```python
from build123d import *

# Parameters (mm, degrees)
F0_R     = 6
F1_DEPTH = 35
F3_DEPTH = 12.5
F5_DEPTH = 25


with BuildPart() as f1:
    # F0 (on Top) → F1 (new body)
    with BuildSketch(Plane.XY):
        Circle(F0_R)
    extrude(amount=F1_DEPTH)

    # F2 (on Front) → F3 (cut, symmetric)
    with BuildSketch(Plane.XZ):
        Polygon((6.1246007681, 35.0653016331), (-6.0470434837, 35.0653016331), (6.1246007681, 22.8936616331), align=None)
    extrude(amount=F3_DEPTH, both=True, mode=Mode.SUBTRACT)

    # F4 (on face) → F5 (join)
    with BuildSketch(Plane(origin=(14.5091301309, 0, 14.5091351992), x_dir=(0.7071069047, 0, -0.7071066577), z_dir=(0.7071066577, 0, 0.7071069047))):
        with BuildLine():
            ThreePointArc((-20.519004735, -6), (-16.2763642357, -4.2426405844), (-14.5190050255, 0))
            ThreePointArc((-14.5190050255, 0), (-16.2763643803, 4.242640729), (-20.519005144, 6))
            ThreePointArc((-20.519005144, 6), (-26.5190050255, -2.045e-07), (-20.519004735, -6))
        make_face()
    extrude(amount=F5_DEPTH)


solid = f1.part
```
Geometry check sheet. Reference: the model listing, model coordinates, mm. Coordinates: 2 decimals unless noted, no trailing zeros. Write each loop counter-clockwise with the first axis right and the second up, starting at its lowest first coordinate (ties: lowest second). Pieces come first, ordered by that corner, then holes. Notation, with made-up numbers: M 49,37.25 L 91,37.25 A28 ccw 91,76.25 Z; hole C -26,50 d2. An arc over 180 degrees is marked long. One line per item, written item: value. Start each with the question number.
(1) Sectioned sample at B-B, the plane z = 9.5. Enter the section's corners in (x, y), and give its area (3 significant figures).
(2) Sectioned sample at A-A, the plane y = -5. Enter the section's corners in (x, z), and give its area (3 significant figures).
(3) Depth check by flat-ended pin: pin 1 (5 mm diameter, centred on y = 0, z = 22, fed in from +X); pin 2 (1 mm diameter, centred on y = -3, z = 9, fed in from -X); pin 3 (4 mm diameter, centred on y = 3, z = 15, fed in from +X). Enter the tip coordinate at first touch or a pass-through.
(4) Release check for a two-part mould opening along X. For faces 1 (the face through (-4.556, -0.472, 33.574)), 2 (the face through (4.54, -0.47, 24.48)), 3 (the face through (0, 0, 0)), 4 (the face through (-6, 0, 13)) record: released by +X, released by -X, zero draft, split by the parting line, or undercut.
(5) Scan lines: line 1 along Z through (x, y) = (-4.5, 0); line 2 along Z through (x, y) = (6.75, 1.5); line 3 along X through (y, z) = (-3, 12.5). Record each from-to range of solid material in increasing order. Write a range as [from, to].
(6) Sectioned sample at C-C, the plane y = 1.5. Enter the section's corners in (x, z), and give its area (3 significant figures).
Filled sheet:
1. outline: C 0,0 d12
1. area: 113 mm²
2. outline: M -3.32,0 L 3.32,0 L 3.32,25.7 L 2.35,26.67 L 20.02,44.35 L 15.33,49.04 L -2.35,31.36 L -3.32,32.33 Z
2. area: 358 mm²
3. pin 1: x = 6
3. pin 2: x = -5.45
3. pin 3: x = 5.92
4. face 1: undercut
4. face 2: released by +X
4. face 3: zero draft
4. face 4: split by the parting line
5. line 1: [0, 33.52]
5. line 2: [27.55, 43.98]
5. line 3: [-5.2, 5.2]
6. outline: M -5.81,0 L 5.81,0 L 5.81,23.21 L 4.11,24.91 L 21.79,42.59 L 13.57,50.8 L -4.11,33.13 L -5.81,34.83 Z
6. area: 628 mm²
